from build123d import *

# Parameters (mm, degrees)
SKETCH1_W                     = 20
SKETCH1_H                     = 95
BASE_FLANGE1_DEPTH            = 0.7366
EDGE_FLANGE1_STRIP_W          = 4.4196
EDGE_FLANGE1_STRIP_H          = 0.7366
EDGE_FLANGE1_STRIP_CUT_DEPTH  = 15
EDGE_FLANGE1_RELIEF_W         = 4.7879
EDGE_FLANGE1_RELIEF_H         = 0.3683
EDGE_FLANGE1_RELIEF_CUT_DEPTH = 0.7366
EDGE_FLANGE1_DEPTH            = 15
EDGE_FLANGE2_STRIP_W          = 4.4196
EDGE_FLANGE2_STRIP_H          = 0.7366
EDGE_FLANGE2_STRIP_CUT_DEPTH  = 15
EDGE_FLANGE2_DEPTH            = 15
EDGE_FLANGE3_STRIP_W          = 4.4196
EDGE_FLANGE3_STRIP_H          = 0.7366
EDGE_FLANGE3_STRIP_CUT_DEPTH  = 15
EDGE_FLANGE3_DEPTH            = 15
EDGE_FLANGE4_STRIP_W          = 4.4196
EDGE_FLANGE4_STRIP_H          = 0.7366
EDGE_FLANGE4_STRIP_CUT_DEPTH  = 15
EDGE_FLANGE4_DEPTH            = 15
SKETCH20_W                    = 18.5268
SKETCH20_H                    = 80
TAB1_DEPTH                    = 0.7366
CUT_EXTRUDE1_DEPTH            = 267.594423465
CUT_EXTRUDE1_DEPTH_BACK       = 267.594423465
SKETCH23_R                    = 1.4
CUT_EXTRUDE2_DEPTH            = 267.594423465
CUT_EXTRUDE2_DEPTH_BACK       = 267.594423465
SKETCH24_R                    = 1.4
FILLET3_R                     = 5
FILLET4_R                     = 5


# Sheet-metal steps are written as plain solids
with BuildPart() as part:
    # Sketch1 → Base-Flange1 (new body)
    with BuildSketch(Plane(origin=(0, 0, 0), x_dir=(1, 0, 0), z_dir=(0, 1, 0))):
        Rectangle(SKETCH1_W, SKETCH1_H)
    extrude(amount=-BASE_FLANGE1_DEPTH)

    # Edge-Flange1 strip (across the edge) → Edge-Flange1 strip cut (cut)
    with BuildSketch(Plane(origin=(10, 0, 47.5), x_dir=(-1, 0, 0), z_dir=(0, 0, -1))):
        with Locations((-1.4732, -0.3683)):
            Rectangle(EDGE_FLANGE1_STRIP_W, EDGE_FLANGE1_STRIP_H)
    extrude(amount=EDGE_FLANGE1_STRIP_CUT_DEPTH, mode=Mode.SUBTRACT)

    # Edge-Flange1 relief (on the sheet) → Edge-Flange1 relief cut (cut)
    with BuildSketch(Plane(origin=(9.2634, 0, 47.5), x_dir=(-1, 0, 0), z_dir=(0, 1, 0))):
        with Locations((-2.02565, -15.18415)):
            Rectangle(EDGE_FLANGE1_RELIEF_W, EDGE_FLANGE1_RELIEF_H)
    extrude(amount=-EDGE_FLANGE1_RELIEF_CUT_DEPTH, mode=Mode.SUBTRACT)

    # Edge-Flange1 section (across the edge) → Edge-Flange1 (add)
    with BuildSketch(Plane(origin=(10, 0, 47.5), x_dir=(-1, 0, 0), z_dir=(0, 0, -1))):
        with BuildLine():
            Line((-0.7366, 0.7366), (-0.7366, 22.2634))
            Line((-0.7366, 22.2634), (0, 22.2634))
            Line((0, 22.2634), (0, 0.7366))
            ThreePointArc((0, 0.7366), (0.215745145, 0.215745145), (0.7366, 0))
            Line((0.7366, 0), (0.7366, -0.7366))
            ThreePointArc((0.7366, -0.7366), (-0.30510971, -0.30510971), (-0.7366, 0.7366))
        make_face()
    extrude(amount=EDGE_FLANGE1_DEPTH)

    # Edge-Flange2 strip (across the edge) → Edge-Flange2 strip cut (cut)
    with BuildSketch(Plane(origin=(10.7366, 22.2634, 32.5), x_dir=(0, -1, 0), z_dir=(0, 0, 1))):
        with Locations((-1.4732, -0.3683)):
            Rectangle(EDGE_FLANGE2_STRIP_W, EDGE_FLANGE2_STRIP_H)
    extrude(amount=EDGE_FLANGE2_STRIP_CUT_DEPTH, mode=Mode.SUBTRACT)

    # Edge-Flange2 section (across the edge) → Edge-Flange2 (add)
    with BuildSketch(Plane(origin=(10.7366, 22.2634, 32.5), x_dir=(0, -1, 0), z_dir=(0, 0, 1))):
        with BuildLine():
            Line((-0.7366, 0.7366), (-0.7366, 134.2634))
            Line((-0.7366, 134.2634), (0, 134.2634))
            Line((0, 134.2634), (0, 0.7366))
            ThreePointArc((0, 0.7366), (0.215745145, 0.215745145), (0.7366, 0))
            Line((0.7366, 0), (0.7366, -0.7366))
            ThreePointArc((0.7366, -0.7366), (-0.30510971, -0.30510971), (-0.7366, 0.7366))
        make_face()
    extrude(amount=EDGE_FLANGE2_DEPTH)

    # Edge-Flange3 strip (across the edge) → Edge-Flange3 strip cut (cut)
    with BuildSketch(Plane(origin=(145, 22.2634, 32.5), x_dir=(-1, 0, 0), z_dir=(0, 0, 1))):
        with Locations((-1.4732, -0.3683)):
            Rectangle(EDGE_FLANGE3_STRIP_W, EDGE_FLANGE3_STRIP_H)
    extrude(amount=EDGE_FLANGE3_STRIP_CUT_DEPTH, mode=Mode.SUBTRACT)

    # Edge-Flange3 section (across the edge) → Edge-Flange3 (add)
    with BuildSketch(Plane(origin=(145, 22.2634, 32.5), x_dir=(-1, 0, 0), z_dir=(0, 0, 1))):
        with BuildLine():
            Line((-0.7366, 0.7366), (-0.7366, 22.2634))
            Line((-0.7366, 22.2634), (0, 22.2634))
            Line((0, 22.2634), (0, 0.7366))
            ThreePointArc((0, 0.7366), (0.215745145, 0.215745145), (0.7366, 0))
            Line((0.7366, 0), (0.7366, -0.7366))
            ThreePointArc((0.7366, -0.7366), (-0.30510971, -0.30510971), (-0.7366, 0.7366))
        make_face()
    extrude(amount=EDGE_FLANGE3_DEPTH)

    # Edge-Flange4 strip (across the edge) → Edge-Flange4 strip cut (cut)
    with BuildSketch(Plane(origin=(145.7366, 0, 47.5), x_dir=(0, 1, 0), z_dir=(0, 0, -1))):
        with Locations((-1.4732, -0.3683)):
            Rectangle(EDGE_FLANGE4_STRIP_W, EDGE_FLANGE4_STRIP_H)
    extrude(amount=EDGE_FLANGE4_STRIP_CUT_DEPTH, mode=Mode.SUBTRACT)

    # Edge-Flange4 section (across the edge) → Edge-Flange4 (add)
    with BuildSketch(Plane(origin=(145.7366, 0, 47.5), x_dir=(0, 1, 0), z_dir=(0, 0, -1))):
        with BuildLine():
            Line((-0.7366, 0.7366), (-0.7366, 19.2634))
            Line((-0.7366, 19.2634), (0, 19.2634))
            Line((0, 19.2634), (0, 0.7366))
            ThreePointArc((0, 0.7366), (0.215745145, 0.215745145), (0.7366, 0))
            Line((0.7366, 0), (0.7366, -0.7366))
            ThreePointArc((0.7366, -0.7366), (-0.30510971, -0.30510971), (-0.7366, 0.7366))
        make_face()
    extrude(amount=EDGE_FLANGE4_DEPTH)

    # Sketch20 → Tab1 (add)
    with BuildSketch(Plane(origin=(0, 0, 0), x_dir=(1, 0, 0), z_dir=(0, 1, 0))):
        with Locations((155.7366, 7.5)):
            Rectangle(SKETCH20_W, SKETCH20_H)
    extrude(amount=-TAB1_DEPTH)

    # Sketch23 → Cut-Extrude1 (cut, two sides: drawn at the far end of the back side and taken through both)
    with BuildSketch(Plane(origin=(10.7366, -49.681752082, -157.421333583), x_dir=(0, 0, -1), z_dir=(1, 0, 0)).offset(-CUT_EXTRUDE1_DEPTH_BACK)):
        with Locations(Location((-199.95707875, 65.413752097, 0), (0, 0, 270))):
            Circle(SKETCH23_R)
    extrude(amount=CUT_EXTRUDE1_DEPTH + CUT_EXTRUDE1_DEPTH_BACK, mode=Mode.SUBTRACT)

    # Sketch24 → Cut-Extrude2 (cut, two sides: drawn at the far end of the back side and taken through both)
    with BuildSketch(Plane(origin=(10.7366, -49.681752082, -157.421333583), x_dir=(0, 0, -1), z_dir=(1, 0, 0)).offset(-CUT_EXTRUDE2_DEPTH_BACK)):
        with Locations(Location((-199.95707875, 55.863752097, 0), (0, 0, 270))):
            Circle(SKETCH24_R)
    extrude(amount=CUT_EXTRUDE2_DEPTH + CUT_EXTRUDE2_DEPTH_BACK, mode=Mode.SUBTRACT)

    # Fillet3
    fillet3_edges = [part.edges().sort_by_distance(p)[0] for p in [
        (-10, -0.3683, 47.5),
    ]]
    fillet(fillet3_edges, radius=FILLET3_R)

    # Fillet4
    fillet4_edges = [part.edges().sort_by_distance(p)[0] for p in [
        (165, -0.3683, 47.5),
    ]]
    fillet(fillet4_edges, radius=FILLET4_R)


solid = part.part
The listing builds one solid part. Answer for the finished solid, in the listing's coordinates (mm). A direction names the side the tool comes from. Round coordinates to 2 decimals unless told otherwise and drop trailing zeros. Write each loop counter-clockwise with the first axis right and the second up, starting at its lowest first coordinate (ties: lowest second). Pieces come first, ordered by that corner, then holes. Notation, with made-up numbers: M 24,5.5 L 53,5.5 A21 cw 53,19.5 Z; hole C -11.75,85.25 d5. An arc over 180 degrees is marked long. Write each question's results on one line, items separated by ' | '. Start each with the question number.
Item 1: A cutting plane is placed at D-D on x = 150. Write down the section's boundary in (y, z).
Item 2: A cutting plane is placed at B-B on y = 10.5. Write down the section's boundary in (x, z), and give its area (3 significant figures).
Item 3: A cutting plane is placed at C-C on z = 37. Write down the section's boundary in (x, y), and give its area (3 significant figures).
Item 4: For faces 1 (the face through (10.737, 11, 40)), 2 (the face through (77.9, 22.6, 47.5)), 3 (the face through (145.737, 11, 40)), 4 (the face through (10, 11, 40)), determine the directions among +Z, -Z, +X, -X, +Y, -Y from which every point of the face is accessible in a straight line to the end or side of a thin tool.
Item 5: Flat-ended cylindrical pins translate along their axes: pin 1 Ø5.5 at (x, z) = (158.5, -21) entering from +Y; pin 2 Ø3 at (y, z) = (6.18, 42.54) entering from +X; pin 3 Ø12 at (x, z) = (79, 38) entering from -Y. Find the tip coordinate at first contact, or state that the pin passes through.
Item 6: A cutting plane is placed at A-A on z = -26.5. Write down the section's boundary in (x, y), and give its area (3 significant figures).
Item 7: For a pull along X with two mould halves and no side action, classify faces 5 (the face through (156, -0.737, -1)), 6 (the face through (-8.5, -0.37, 46.07)), 7 (the face through (145, 11, 40)) as pulls with the +X half, pulls with the -X half, needs draft (parallel to the pull), parting line crosses it, or undercut.
Item 8: Straight lines are drawn through the part: L1, parallel to X at y = 7.25, z = 40.5; L2, parallel to Y at x = 147.5, z = 23. For each, find the intervals that lie inside material, in ascending order. Write a range as [from, to].
Check sheet entries:
1) outline: M -0.74,-47.5 L 0,-47.5 L 0,47.5 L -0.74,47.5 Z
2) outline: M 10,32.5 L 10.74,32.5 L 10.74,47.5 L 10,47.5 Z; M 145,32.5 L 145.74,32.5 L 145.74,47.5 L 145,47.5 Z | area: 22.1 mm²
3) outline: M -10,-0.74 L 9.26,-0.74 A1.47 ccw 10.74,0.74 L 10.74,21.53 A0.74 cw 11.47,22.26 L 144.26,22.26 A0.74 cw 145,21.53 L 145,0.74 A1.47 ccw 146.47,-0.74 L 165,-0.74 L 165,0 L 146.47,0 A0.74 cw 145.74,0.74 L 145.74,21.53 A1.47 ccw 144.26,23 L 11.47,23 A1.47 ccw 10,21.53 L 10,0.74 A0.74 cw 9.26,0 L -10,0 Z | area: 161 mm²
4) face 1: +Z, -Z, -Y | face 2: +Z, +X, -X, +Y, -Y | face 3: +Z, -Z, +X, +Y | face 4: +Z, -Z, -X, +Y
5) pin 1: y = 0 | pin 2: x = 145.74 | pin 3: y = 22.26
6) outline: M -10,-0.74 L 10,-0.74 L 10,0 L -10,0 Z; M 146.47,-0.74 L 165,-0.74 L 165,0 L 146.47,0 Z | area: 28.4 mm²
7) face 5: needs draft | face 6: pulls with the -X half | face 7: undercut
8) L1: [10, 10.74], [145, 145.74] | L2: [-0.74, 0]
